```python
from build123d import *

# Parameters (mm, degrees)
SKETCH1_R              = 1.6
ARDUINO_TEMPLATE_DEPTH = 1


with BuildPart() as part:
    # Sketch1 → Arduino Template (new body)
    # profile 1 of 3: a face of its own
    with BuildSketch(Plane(origin=(0, 0, 0), x_dir=(1, 0, 0), z_dir=(0, 1, 0))):
        Polygon((101.61, 3.81), (101.61, 38.09), (97.8, 38.09), (97.8, 41.9), (97.8, 49.52), (93.99, 53.33), (0, 53.33), (0, 0), (97.8, 0), (98.9, 1.1), align=None)
        with Locations(Location((14, 2.5, 0), (0, 0, 270))):
            Circle(SKETCH1_R, mode=Mode.SUBTRACT)
        with Locations(Location((66.1, 7.6, 0), (0, 0, 270))):
            Circle(SKETCH1_R, mode=Mode.SUBTRACT)
        with Locations(Location((96.53, 2.5, 0), (0, 0, 270))):
            Circle(SKETCH1_R, mode=Mode.SUBTRACT)
        with Locations(Location((15.3, 50.83, 0), (0, 0, 270))):
            Circle(SKETCH1_R, mode=Mode.SUBTRACT)
        with Locations(Location((66.1, 35.5, 0), (0, 0, 270))):
            Circle(SKETCH1_R, mode=Mode.SUBTRACT)
        with Locations(Location((90.2, 50.83, 0), (0, 0, 270))):
            Circle(SKETCH1_R, mode=Mode.SUBTRACT)
    # profile 2 of 3: a face of its own
    with BuildSketch(Plane(origin=(0, 0, 0), x_dir=(1, 0, 0), z_dir=(0, 1, 0))):
        Polygon((98.9, 0), (98.9, 1.1), (97.8, 0), align=None)
    # profile 3 of 3: a face of its own
    with BuildSketch(Plane(origin=(0, 0, 0), x_dir=(1, 0, 0), z_dir=(0, 1, 0))):
        Polygon((97.8, 38.09), (101.61, 38.09), (97.8, 41.9), align=None)
    extrude(amount=ARDUINO_TEMPLATE_DEPTH)


solid = part.part
```
Model file for the job. Use its own axes, mm. Give positions to 0.01 mm unless a question says otherwise; leave off trailing zeros. Write each loop counter-clockwise with the first axis right and the second up, starting at its lowest first coordinate (ties: lowest second). Pieces come first, ordered by that corner, then holes. Notation, with made-up numbers: (16, 40) -> (47, 40) arc R13 ccw to (47, 65) -> close; hole circle Ø3 at (66.25, 76). An arc over 180 degrees is marked (long way). Use CSV: the item, a comma, the result in double quotes. Start each with the question number.
1) Cut at B-B on x = 96.53. List the corners of the cut face in (y, z), plus the area to 3 significant figures.
2) Cut at A-A on z = -7.6. List the corners of the cut face in (x, y).
3) Two-plate mould, pull along X, no slides. Class faces 1 (the flat face through (95.92, 0.49, -51.4)), 2 (the flat face through (50, 0, -27)), 3 (the cylindrical face through (64.54, 0.49, -35.85)): released by +X, released by -X, zero draft, split by the parting line, or undercut.
4) Cut at C-C on y = 0.8. List the corners of the cut face in (x, z), plus the area to 3 significant figures.
5) Cut at D-D on z = -50.83. List the corners of the cut face in (x, y).
6) Drill centre lines: L1, parallel to Z at x = 66.1, y = 0.6; L2, parallel to X at y = 0.2, z = -7.6; L3, parallel to Z at x = 66.5, y = 0.85. Where is each one in solid material? Low to high.
Final values:
1,outline,"(0, -50.79) -> (1, -50.79) -> (1, -4.1) -> (0, -4.1) -> close; (0, -0.9) -> (1, -0.9) -> (1, 0) -> (0, 0) -> close"
1,area,"47.6 mm2"
2,outline,"(0, 0) -> (64.5, 0) -> (64.5, 1) -> (0, 1) -> close; (67.7, 0) -> (101.61, 0) -> (101.61, 1) -> (67.7, 1) -> close"
3,face 1,"released by +X"
3,face 2,"zero draft"
3,face 3,"undercut"
4,outline,"(0, -53.33) -> (93.99, -53.33) -> (97.8, -49.52) -> (97.8, -41.9) -> (101.61, -38.09) -> (101.61, -3.81) -> (98.9, -1.1) -> (98.9, 0) -> (0, 0) -> close; hole circle Ø3.2 at (14, -2.5); hole circle Ø3.2 at (15.3, -50.83); hole circle Ø3.2 at (66.1, -35.5); hole circle Ø3.2 at (66.1, -7.6); hole circle Ø3.2 at (90.2, -50.83); hole circle Ø3.2 at (96.53, -2.5)"
4,area,"5,310 mm2"
5,outline,"(0, 0) -> (13.7, 0) -> (13.7, 1) -> (0, 1) -> close; (16.9, 0) -> (88.6, 0) -> (88.6, 1) -> (16.9, 1) -> close; (91.8, 0) -> (96.49, 0) -> (96.49, 1) -> (91.8, 1) -> close"
6,L1,"z = -53.33 to -37.1, -33.9 to -9.2, -6 to 0"
6,L2,"x = 0 to 64.5, 67.7 to 101.61"
6,L3,"z = -53.33 to -37.05, -33.95 to -9.15, -6.05 to 0"
